Design review of the part built by this model. Coordinates are the model's own, in mm. Face numbers are marked on the shaded views. A direction names the side the tool comes from. Round coordinates to 2 decimals unless told otherwise and drop trailing zeros. Write each loop counter-clockwise with the first axis right and the second up, starting at its lowest first coordinate (ties: lowest second). Pieces come first, ordered by that corner, then holes. Notation, with made-up numbers: (16.5, 89) -> (49.5, 89) arc R34 cw to (49.5, 124) -> close; hole circle Ø8 at (-3, 49.25). An arc over 180 degrees is marked (long way). Write item = value, one per line. Start each with the question number.
Item 1: Add section B-B, the plane x = 10.5. State the section outline as (y, z) points, then the cut area to 3 significant figures.
Item 2: Mouldability with a two-part tool opening along X and no side actions: class the marked faces 3, 4 and 5 as released by +X, released by -X, zero draft, split by the parting line, or undercut.
Item 3: Add section C-C, the plane y = 4. State the section outline as (x, z) points (3 decimals), then the cut area to 3 significant figures.
Item 4: To check wall thickness, follow L1, parallel to Y at x = -37, z = -30; L2, parallel to X at y = 13, z = -71; L3, parallel to X at y = 16, z = 13.5. State the ranges of each line that lie inside material, in increasing order.
Item 5: Add section A-A, the plane z = 0. State the section outline as (x, y) points (3 decimals).
Item 6: For pin 1 Ø11 at (x, y) = (0, 36.83) entering from -Z; pin 2 Ø14.5 at (x, z) = (-54.35, -17.66) entering from +Y; pin 3 Ø1.5 at (x, y) = (6, 19) entering from -Z, all flat-tipped, find the tip position at first contact; note any pin that passes through.
Item 7: Machinability: for the marked faces 1 and 2, which of the approach directions +Z, -Z, +X, -X, +Y, -Y give a long, thin tool a straight path to every point of the face, cutting with its end or side? Answer none if there is none.
from build123d import *

# Parameters (mm, degrees)
SKETCH1_W                  = 17.145
SKETCH1_H                  = 31.75
SKETCH1_W_2                = 69.85
SKETCH1_H_2                = 15.24
F_1_2_0_5_DIAMETER_HOLE1_D = 12.7
CUT_EXTRUDE1_DEPTH         = 131.021580324
CUT_EXTRUDE1_DEPTH_BACK    = 131.021580324
SKETCH10_R                 = 4.7625


with BuildPart() as part:
    # Sketch1 → Revolve1 (revolve)
    with BuildSketch(Plane.XY, mode=Mode.PRIVATE) as revolve1_sk:
        with Locations((24.4475, 31.115)):
            Rectangle(SKETCH1_W, SKETCH1_H)
        with Locations((50.8, 7.62)):
            Rectangle(SKETCH1_W_2, SKETCH1_H_2)
    revolve(revolve1_sk.sketch.rotate(Axis((0, 7.809475806, 0), (0, -1, 0)), 90), axis=Axis((0, 7.809475806, 0), (0, -1, 0)))

    # 1/2 (0.5) Diameter Hole1 (through all)
    with Locations(Plane(origin=(0, 15.24, 0), x_dir=(1, 0, 0), z_dir=(0, 1, 0))):
        with Locations((-54.352879906, 17.660321229), (0, 57.15), (54.352879906, 17.660321229), (33.591927169, -46.235321229), (-33.591927169, -46.235321229)):
            Hole(F_1_2_0_5_DIAMETER_HOLE1_D / 2)

    # Sketch10 → Cut-Extrude1 (cut, two sides: drawn at the far end of the back side and taken through both)
    with BuildSketch(Plane.XY.offset(-CUT_EXTRUDE1_DEPTH_BACK)):
        with Locations((0, 36.83)):
            Circle(SKETCH10_R)
    extrude(amount=CUT_EXTRUDE1_DEPTH + CUT_EXTRUDE1_DEPTH_BACK, mode=Mode.SUBTRACT)


solid = part.part
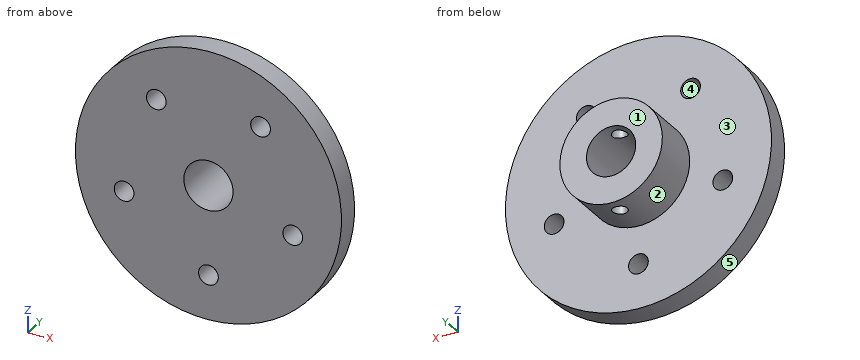
Result set:
q1.outline = (0, -85.08) -> (15.24, -85.08) -> (15.24, -31.31) -> (46.99, -31.31) -> (46.99, -11.91) -> (0, -11.91) -> close; (0, 11.91) -> (46.99, 11.91) -> (46.99, 31.31) -> (15.24, 31.31) -> (15.24, 85.08) -> (0, 85.08) -> close
q1.area = 3,460 mm²
q2.face_3 = zero draft
q2.face_4 = undercut
q2.face_5 = split by the parting line
q3.outline = circle Ø171.45 at (0, 0); hole circle Ø12.7 at (-54.353, -17.66); hole circle Ø12.7 at (-33.592, 46.235); hole circle Ø31.75 at (0, 0); hole circle Ø12.7 at (0, -57.15); hole circle Ø12.7 at (33.592, 46.235); hole circle Ø12.7 at (54.353, -17.66)
q3.area = 21,700 mm²
q4.L1 = 0 to 15.24
q4.L2 = -48.04 to 48.04
q4.L3 = -30.13 to -8.35, 8.35 to 30.13
q5.outline = (-85.725, 0) -> (-15.875, 0) -> (-15.875, 46.99) -> (-33.02, 46.99) -> (-33.02, 15.24) -> (-85.725, 15.24) -> close; (15.875, 0) -> (85.725, 0) -> (85.725, 15.24) -> (33.02, 15.24) -> (33.02, 46.99) -> (15.875, 46.99) -> close
q6.pin_1 = -33.02
q6.pin_2 = 15.24
q6.pin_3 = -32.6
q7.face_1 = +Z, -Z, +X, -X, +Y
q7.face_2 = +Y
